The model under review builds one solid part; all positions refer to its coordinate system, in mm. A direction names the side the tool comes from. Round coordinates to 2 decimals unless told otherwise and drop trailing zeros. Order: outer loops, then holes, each group sorted by start corner. A loop starts at its lowest first (then second) coordinate and runs counter-clockwise, first axis right, second up.
1) Consider section D-D (y = 7). Give the boundary of the cut face in (x, z) (3 decimals), then the cut area to 3 significant figures.
2) Clearance check with flat-ended pins moving along their axes: P1, Ø1.5, axis at y = -24, z = 4, coming from the -X side; P2, Ø2, axis at x = 63, z = 3, coming from the -Y side; P3, Ø2, axis at y = -13.5, z = 4, coming from the +X side. State where each tip first meets the part, or that it passes through.
3) Consider section C-C (z = 2.25). Give the number of separate pieces and of enclosed holes in the cut face, then the cut area to 3 significant figures.
4) Consider section B-B (x = 7). Give the boundary of the cut face in (y, z) (3 decimals), then the cut area to 3 significant figures.
5) To check wall thickness, follow L1, parallel to X at y = -26, z = 2.8; L2, parallel to Y at x = 0, z = 1.3 (3 decimals); L3, parallel to X at y = -29, z = 4.6. State the ranges of each line that lie inside material, in increasing order.
6) Machinability: for faces 1 (the face through (43.525, -5.167, 2.465)), 2 (the face through (33.601, -28.113, 2.465)), 3 (the face through (67.771, -12.968, 2.465)), which of the approach directions +Z, -Z, +X, -X, +Y, -Y give a long, thin tool a straight path to every point of the face, cutting with its end or side? Answer none if there is none.
7) Consider section A-A (y = 0). Give the boundary of the cut face in (x, z) (3 decimals), then the cut area to 3 significant figures.
8) Mouldability with a two-part tool opening along Y and no side actions: class faces 4 (the face through (23.514, 0.725, 2.465)), 5 (the face through (0.59, -8.13, 2.46)), 6 (the face through (39, -20, 5)) as pulls with the +Y half, pulls with the -Y half, needs draft (parallel to the pull), parting line crosses it, or undercut.
from build123d import *

# Parameters (mm, degrees)
ESQUISSE2_R        = 1.275
ESQUISSE2_R_2      = 3
BOSS_EXTRU_1_DEPTH = 5


with BuildPart() as part:
    # Esquisse2 → Boss.-Extru.1 (new body)
    with BuildSketch(Plane.XY):
        with BuildLine():
            Line((42.518708235, -7.493960905), (3.969600002, 9.178359103))
            ThreePointArc((3.969600002, 9.178359103), (-9.178359103, 3.969600002), (-3.969600002, -9.178359103))
            Line((-3.969600002, -9.178359103), (34.579508231, -25.850679111))
            Line((34.579508231, -25.850679111), (32.59470823, -30.439858662))
            Line((32.59470823, -30.439858662), (78.486503746, -50.287858671))
            Line((78.486503746, -50.287858671), (90.395303751, -22.752781362))
            Line((90.395303751, -22.752781362), (44.503508236, -2.904781353))
            Line((44.503508236, -2.904781353), (42.518708235, -7.493960905))
        make_face()
        with Locations((7, 0)):
            Circle(ESQUISSE2_R, mode=Mode.SUBTRACT)
        with Locations((0, 7)):
            Circle(ESQUISSE2_R, mode=Mode.SUBTRACT)
        with Locations((-7, 0)):
            Circle(ESQUISSE2_R, mode=Mode.SUBTRACT)
        with Locations((0, -7)):
            Circle(ESQUISSE2_R, mode=Mode.SUBTRACT)
        with Locations((75.882124195, -43.713879119)):
            Circle(ESQUISSE2_R_2, mode=Mode.SUBTRACT)
        with Locations((83.821324199, -25.357160913)):
            Circle(ESQUISSE2_R_2, mode=Mode.SUBTRACT)
        with Locations((47.107887786, -9.478760905)):
            Circle(ESQUISSE2_R_2, mode=Mode.SUBTRACT)
        with Locations((39.168687783, -27.835479112)):
            Circle(ESQUISSE2_R_2, mode=Mode.SUBTRACT)
    extrude(amount=BOSS_EXTRU_1_DEPTH)


solid = part.part
Answer below:
1. outline: (-7.141, 0) - (-1.275, 0) - (-1.275, 5) - (-7.141, 5) - close; (1.275, 0) - (9.006, 0) - (9.006, 5) - (1.275, 5) - close
1. area: 68.0 mm2
2. P1: stops at x = 28.57
2. P2: stops at y = -44.02
2. P3: stops at x = 71.31
3. separate pieces: 1
3. enclosed holes: 8
3. area: 2,360 mm2
4. outline: (-13.923, 0) - (-1.275, 0) - (-1.275, 5) - (-13.923, 5) - close; (1.275, 0) - (7.868, 0) - (7.868, 5) - (1.275, 5) - close
4. area: 96.2 mm2
5. L1: x = 34.51 to 36.8, 41.54 to 80.89, 86.75 to 88.99
5. L2: y = -10.895 to -8.275, -5.725 to 5.725, 8.275 to 10
5. L3: x = 33.22 to 36.4, 41.93 to 87.69
6. face 1: +Z, -Z, +Y
6. face 2: +Z, -Z, -X
6. face 3: +Z, -Z, +X, +Y
7. outline: (-10, 0) - (-8.275, 0) - (-8.275, 5) - (-10, 5) - close; (-5.725, 0) - (5.725, 0) - (5.725, 5) - (-5.725, 5) - close; (8.275, 0) - (25.191, 0) - (25.191, 5) - (8.275, 5) - close
7. area: 150 mm2
8. face 4: pulls with the +Y half
8. face 5: undercut
8. face 6: needs draft
